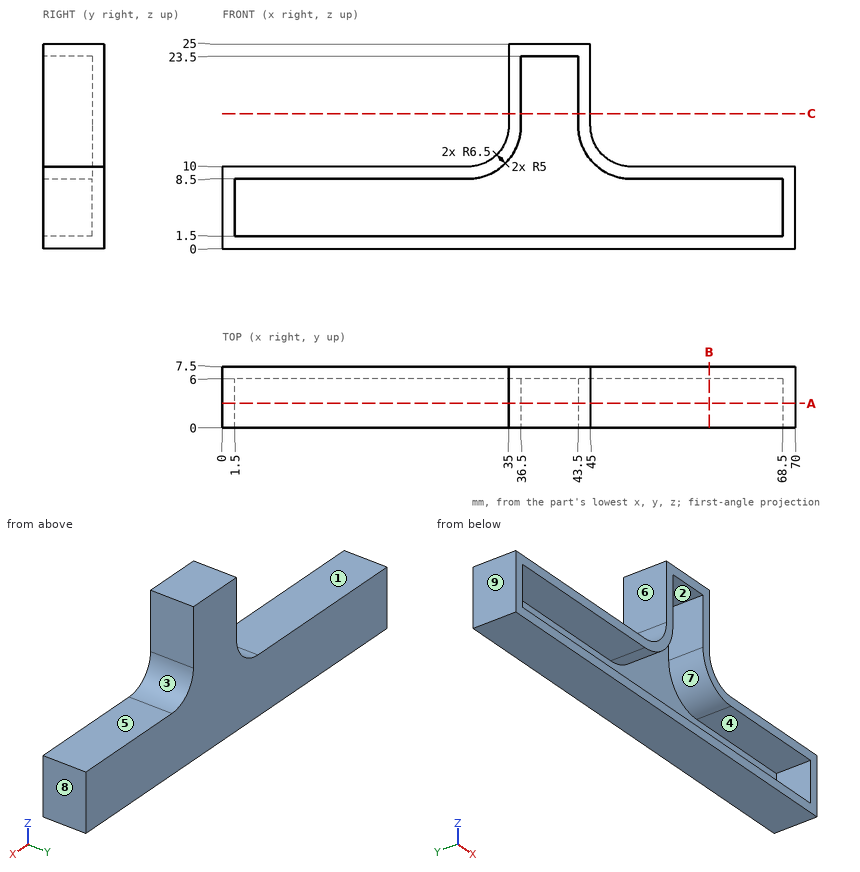
Geometry check sheet. Reference: drawing and pictorial views, mm from the part's lowest x, y, z. A direction names the side the tool comes from. Coordinates: 2 decimals unless noted, no trailing zeros. Order: outer loops, then holes, each group sorted by start corner. A loop starts at its lowest first (then second) coordinate and runs counter-clockwise, first axis right, second up.
Item 1: Tool access check on the marked faces 5, 6, 7, 8 and 9. Record the directions out of +Z, -Z, +X, -X, +Y, -Y that give a thin tool (end or side, any length) a straight path to the whole face; none if there is none.
Item 2: Section check C-C (z = 16.5). Enter the section's corners in (x, y).
Item 3: Mould release check, pull along X, two halves, no side actions. Record for the marked faces 1, 2, 3 and 4: released by +X, released by -X, zero draft, split by the parting line, or undercut.
Item 4: Section check A-A (y = 3). Enter the section's corners in (x, z), plus the area to 3 significant figures.
Item 5: Depth check by flat-ended pin: pin 1 (4 mm diameter, centred on y = 3.5, z = 21.5, fed in from -X); pin 2 (4 mm diameter, centred on y = 2, z = 12.5, fed in from +X); pin 3 (4 mm diameter, centred on x = 14.5, y = 4.5, fed in from +Z). Enter the tip coordinate at first touch or a pass-through.
Item 6: Scan lines: line 1 along Z through (x, y) = (29, 1.5); line 2 along X through (y, z) = (5.5, 7.5); line 3 along X through (y, z) = (5, 18). Record each from-to range of solid material in increasing order.
Item 7: Section check B-B (x = 59.5). Enter the section's corners in (y, z), plus the area to 3 significant figures.
Check sheet entries:
1. face 5: +Z, +X, +Y, -Y
1. face 6: +Z, -X, +Y, -Y
1. face 7: -Y
1. face 8: +Z, -Z, +X, +Y, -Y
1. face 9: +Z, -Z, -X, +Y, -Y
2. outline: (35, 0) - (36.5, 0) - (36.5, 6) - (43.5, 6) - (43.5, 0) - (45, 0) - (45, 7.5) - (35, 7.5) - close
3. face 1: zero draft
3. face 2: undercut
3. face 3: released by +X
3. face 4: undercut
4. outline: (0, 0) - (70, 0) - (70, 10) - (50, 10) arc R5 cw to (45, 15) - (45, 25) - (35, 25) - (35, 15) arc R5 cw to (30, 10) - (0, 10) - close; hole (1.5, 1.5) - (68.5, 1.5) - (68.5, 8.5) - (50, 8.5) arc R6.5 cw to (43.5, 15) - (43.5, 23.5) - (36.5, 23.5) - (36.5, 15) arc R6.5 cw to (30, 8.5) - (1.5, 8.5) - close
4. area: 269 mm2
5. pin 1: stops at x = 35
5. pin 2: stops at x = 47.82
5. pin 3: stops at z = 10
6. line 1: z = 0 to 1.5, 8.5 to 10
6. line 2: x = 0 to 1.5, 68.5 to 70
6. line 3: x = 35 to 36.5, 43.5 to 45
7. outline: (0, 0) - (7.5, 0) - (7.5, 10) - (0, 10) - (0, 8.5) - (6, 8.5) - (6, 1.5) - (0, 1.5) - close
7. area: 33.0 mm2
